The figure shows three views and two pictorial views of one solid part (mm, origin at its lowest corner). Answer the questions. A direction names the side the tool comes from. Coordinates: 2 decimals unless noted, no trailing zeros. Write each loop counter-clockwise with the first axis right and the second up, starting at its lowest first coordinate (ties: lowest second). Pieces come first, ordered by that corner, then holes. Notation, with made-up numbers: (9, -20) - (48, -20) arc R32 cw to (48, 6) - close; hole circle Ø5 at (31, 30). An arc over 180 degrees is marked (long way). Use a Markdown table: item, result. Add a question column.
(1) The part is cut by section C-C, the plane y = 39. Give the vertices of the cut face in (x, z), then the cut area to 3 significant figures.
(2) The part is cut by section A-A, the plane y = 18.5. Give the vertices of the cut face in (x, z).
(3) The part is cut by section B-B, the plane z = 2. Give the vertices of the cut face in (x, y).
(4) The part is cut by section D-D, the plane x = 32.5. Give the vertices of the cut face in (y, z), then the cut area to 3 significant figures.
(5) For a pull along X with two mould halves and no side action, classify the marked faces 1, 2, 3 and 4 as released by +X, released by -X, zero draft, split by the parting line, or undercut.
(6) Find the intervals of material crossed by line 1 (X direction, y = 19, z = 1); line 2 (Z direction, x = 19, y = 22.5); line 3 (X direction, y = 16, z = 3.75), in increasing order. Write a range as from..to.
(7) A tool of negligible diameter and unlimited length cuts with its end or side. For the marked faces 5 and 6, from which of +Z, -Z, +X, -X, +Y, -Y can it reach the whole face along a straight path? Write none if from no direction.
(8) Given pin 1 Ø1 at (y, z) = (14.5, 6.5) entering from -X; pin 2 Ø6 at (x, y) = (9.5, 10.5) entering from +Z; pin 3 Ø0.6 at (y, z) = (14, 7) entering from +X, each flat-ended and moving along its own axis, determine where each tip first touches the part or whether it passes through.
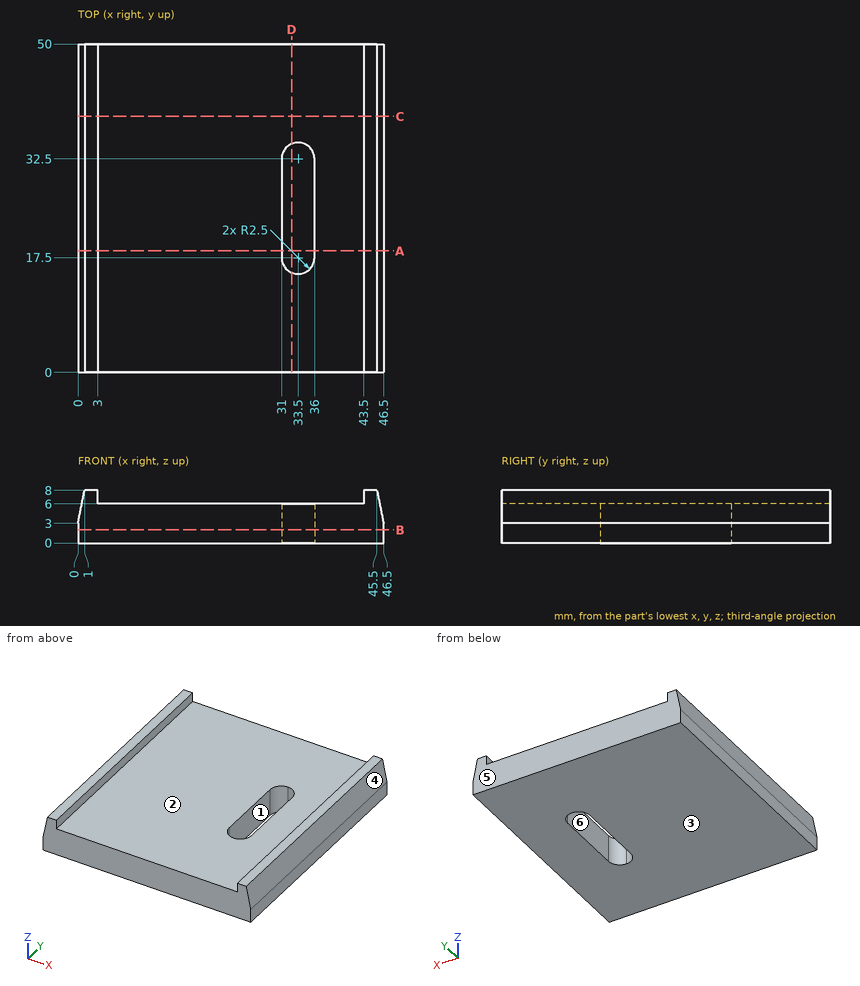
Model answer:
| question | item | result |
|---|---|---|
| 1 | outline | (0, 0) - (46.5, 0) - (46.5, 3) - (45.5, 8) - (43.5, 8) - (43.5, 6) - (3, 6) - (3, 8) - (1, 8) - (0, 3) - close |
| 1 | area | 286 mm^2 |
| 2 | outline | (0, 0) - (31, 0) - (31, 6) - (3, 6) - (3, 8) - (1, 8) - (0, 3) - close; (36, 0) - (46.5, 0) - (46.5, 3) - (45.5, 8) - (43.5, 8) - (43.5, 6) - (36, 6) - close |
| 3 | outline | (0, 0) - (46.5, 0) - (46.5, 50) - (0, 50) - close; hole (31, 17.5) arc R2.5 ccw to (36, 17.5) - (36, 32.5) arc R2.5 ccw to (31, 32.5) - close |
| 4 | outline | (0, 0) - (15.21, 0) - (15.21, 6) - (0, 6) - close; (34.79, 0) - (50, 0) - (50, 6) - (34.79, 6) - close |
| 4 | area | 183 mm^2 |
| 5 | face 1 | undercut |
| 5 | face 2 | undercut |
| 5 | face 3 | zero draft |
| 5 | face 4 | released by +X |
| 6 | line 1 | 0..31, 36..46.5 |
| 6 | line 2 | 0..6 |
| 6 | line 3 | 0.15..31.5, 35.5..46.35 |
| 7 | face 5 | +Z, -Z, +X, -X, +Y |
| 7 | face 6 | +Z, -Z |
| 8 | pin 1 | x = 0.6 |
| 8 | pin 2 | z = 6 |
| 8 | pin 3 | x = 45.76 |
